Read the model definition and answer for the solid it produces. Units are mm, in the model's axes. A direction names the side the tool comes from. Give positions to 0.01 mm unless a question says otherwise; leave off trailing zeros. Write each loop counter-clockwise with the first axis right and the second up, starting at its lowest first coordinate (ties: lowest second). Pieces come first, ordered by that corner, then holes. Notation, with made-up numbers: (36.25, 17.25) - (60.25, 17.25) arc R18 ccw to (60.25, 28.25) - close; hole circle Ø5 at (-4, 19). An arc over 180 degrees is marked (long way). Answer as CSV lines item,"result".
```python
from build123d import *

# Parameters (mm, degrees)
F0_R     = 1.5
F1_DEPTH = 2
F2_W     = 3
F2_H     = 7.5
F3_DEPTH = 3
F4_DEPTH = 5.5
F5_R     = 2


# Not quite as in the source:
# - a pattern or mirror of a feature is missing from the dataset's text; its kind, count and spacing are read off the source's solid


with BuildPart() as f1:
    # F0 (on Top) → F1 (new body)
    with BuildSketch(Plane.XY):
        Polygon((12.5, 12), (0, 12), (-12.5, 12), (-12.5, -3), (-10, -3), (-10, -12), (0, -12), (10, -12), (10, -3), (12.5, -3), align=None)
        with Locations((0, 4.5)):
            Circle(F0_R, mode=Mode.SUBTRACT)
    extrude(amount=F1_DEPTH)

    # F2 (on face) → F3 (join)
    with BuildSketch(Plane.XY.offset(2)):
        with Locations((8.5, -8.25)):
            Rectangle(F2_W, F2_H)
    f3 = extrude(amount=F3_DEPTH)

    # F3_copies: F3 across plane
    add(f3.mirror(Plane(origin=(0, 0, 0), x_dir=(0, 0, -1), z_dir=(-1, 0, 0))))

    # F2 (on face) → F4 (join)
    with BuildSketch(Plane.XY.offset(2)):
        with Locations((11, 5.25)):
            Rectangle(F2_W, F2_H)
    f4 = extrude(amount=F4_DEPTH)

    # F4_copies: F4 across plane
    add(f4.mirror(Plane(origin=(0, 0, 0), x_dir=(0, 0, -1), z_dir=(-1, 0, 0))))

    # F5
    f5_edges = [f1.edges().sort_by_distance(p)[0] for p in [
        (12.5, 12, 1),
        (12.5, -3, 1),
        (-12.5, -3, 1),
        (-12.5, 12, 1),
    ]]
    fillet(f5_edges, radius=F5_R)


solid = f1.part
```
(1) Each of these flat-tipped pins is pushed along its axis until it touches: P1, Ø1.5, axis at x = -9, z = 4, coming from the +Y side; P2, Ø2.5, axis at y = -9.5, z = 4, coming from the -X side; P3, Ø2, axis at x = 2, y = -1, coming from the +Z side; P4, Ø2, axis at x = 5, z = 4.5, coming from the +Y side. Where does it stop, or does it pass through?
Worked out:
P1,"stops at y = 9"
P2,"stops at x = -10"
P3,"stops at z = 2"
P4,"passes through"
(2) A cutting plane is placed at C-C (x = 0). Write down the section's boundary in (y, z), and give its area (3 significant figures).
Worked out:
outline,"(-12, 0) - (3, 0) - (3, 2) - (-12, 2) - close; (6, 0) - (12, 0) - (12, 2) - (6, 2) - close"
area,"42.0 mm^2"
(3) For faces 1 (the flat face through (-10, -8, 2)), 2 (the flat face through (7, -8, 3)), 3 (the flat face through (11, 1.5, 5)), 4 (the flat face through (-11, 9, 5)), determine the directions among +Z, -Z, +X, -X, +Y, -Y from which every point of the face is accessible in a straight line to the end or side of a thin tool.
Worked out:
face 1,"+Z, -Z, -X, -Y"
face 2,"+Z, +Y, -Y"
face 3,"+Z, +X, -X"
face 4,"+Z, +X, -X, +Y"
(4) The mould has two halves that part along X. Classify faces 5 (the flat face through (0, 12, 1)), 6 (the flat face through (10, -8, 2)), 7 (the flat face through (9.5, 5, 5)): +X half, -X half, draft (parallel to the pull), parting line (faces both ways), or undercut.
Worked out:
face 5,"draft"
face 6,"+X half"
face 7,"undercut"
(5) A cutting plane is placed at D-D (y = -8.5). Write down the section's boundary in (x, z).
Worked out:
outline,"(-10, 0) - (10, 0) - (10, 5) - (7, 5) - (7, 2) - (-7, 2) - (-7, 5) - (-10, 5) - close"
(6) A cutting plane is placed at A-A (y = 4.5). Write down the section's boundary in (x, z), and give its area (3 significant figures).
Worked out:
outline,"(-12.5, 0) - (-1.5, 0) - (-1.5, 2) - (-9.5, 2) - (-9.5, 7.5) - (-12.5, 7.5) - close; (1.5, 0) - (12.5, 0) - (12.5, 7.5) - (9.5, 7.5) - (9.5, 2) - (1.5, 2) - close"
area,"77.0 mm^2"
(7) A cutting plane is placed at B-B (z = 4.5). Write down the section's boundary in (x, y), and give its area (3 significant figures).
Worked out:
outline,"(-12.5, 1.5) - (-9.5, 1.5) - (-9.5, 9) - (-12.5, 9) - close; (-10, -12) - (-7, -12) - (-7, -4.5) - (-10, -4.5) - close; (7, -12) - (10, -12) - (10, -4.5) - (7, -4.5) - close; (9.5, 1.5) - (12.5, 1.5) - (12.5, 9) - (9.5, 9) - close"
area,"90.0 mm^2"
(8) Find the intervals of material crossed by L1, parallel to Y at x = 0, z = 1.6; L2, parallel to X at y = 8.75, z = 6.75; L3, parallel to Z at x = 7, y = 4.5, in increasing order.
Worked out:
L1,"y = -12 to 3, 6 to 12"
L2,"x = -12.5 to -9.5, 9.5 to 12.5"
L3,"z = 0 to 2"
